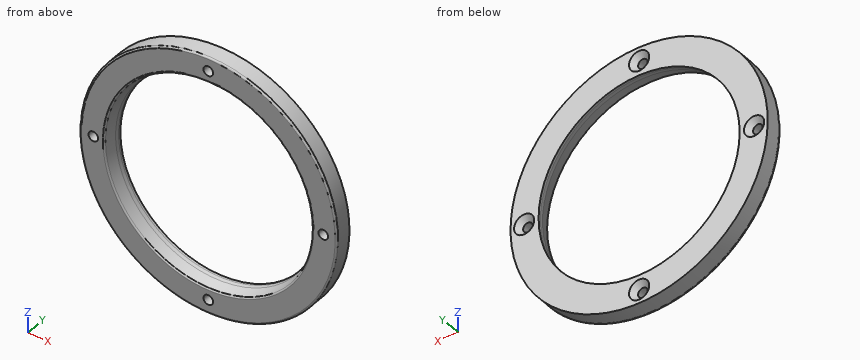
```python
from build123d import *

# Parameters (mm, degrees)
SKETCH1_R                                       = 59.944
SKETCH1_R_2                                     = 47.244
BOSS_EXTRUDE1_DEPTH                             = 8.128
CSK_FOR_M4_FLAT_HEAD_MACHINE_SCREW1_D           = 4.5
CSK_FOR_M4_FLAT_HEAD_MACHINE_SCREW1_CSINK_D     = 9.4
CSK_FOR_M4_FLAT_HEAD_MACHINE_SCREW1_CSINK_ANGLE = 90
CIRPATTERN1_COUNT                               = 4
DRAFT2_ANGLE                                    = 15
SKETCH5_R                                       = 46.865275631
CUT_EXTRUDE1_DEPTH                              = 86.162378173
FILLET1_R                                       = 6.35
FILLET2_R                                       = 0.79375


with BuildPart() as part:
    # Sketch1 → Boss-Extrude1 (new body)
    with BuildSketch(Plane(origin=(0, 0, 0), x_dir=(1, 0, 0), z_dir=(0, 1, 0))):
        with Locations(Location((0, 0, 0), (0, 0, 270))):
            Circle(SKETCH1_R)
        with Locations(Location((0, 0, 0), (0, 0, 270))):
            Circle(SKETCH1_R_2, mode=Mode.SUBTRACT)
    extrude(amount=BOSS_EXTRUDE1_DEPTH)

    # CSK for M4 Flat Head Machine Screw1 (through all)
    with Locations(Plane(origin=(0, 8.128, -53.594), x_dir=(0, 0, 1), z_dir=(0, 1, 0))):
        with Locations((0, 0)):
            csk_for_m4_flat_head_machine_screw1 = CounterSinkHole(CSK_FOR_M4_FLAT_HEAD_MACHINE_SCREW1_D / 2, CSK_FOR_M4_FLAT_HEAD_MACHINE_SCREW1_CSINK_D / 2, counter_sink_angle=CSK_FOR_M4_FLAT_HEAD_MACHINE_SCREW1_CSINK_ANGLE)

    # CirPattern1: CSK for M4 Flat Head Machine Screw1 ×4 about axis
    cirpattern1_axis = Axis((0, 0, 0), (0, 1, 0))
    for i in range(1, CIRPATTERN1_COUNT):
        add(csk_for_m4_flat_head_machine_screw1.rotate(cirpattern1_axis, i * 360 / CIRPATTERN1_COUNT), mode=Mode.SUBTRACT)

    # Draft2
    draft2_faces = [part.faces().sort_by_distance(p)[0] for p in [
        (0, 4.064, -47.244),
    ]]
    draft(draft2_faces, Plane(origin=(0, 0, 0), x_dir=(0, 0, -1), z_dir=(0, -1, 0)), DRAFT2_ANGLE)

    # Sketch4 → Cut-Revolve1 (revolve, cut)
    with BuildSketch(Plane(origin=(0, 0, 0), x_dir=(0, 0, -1), z_dir=(1, 0, 0)), mode=Mode.PRIVATE) as cut_revolve1_sk:
        Polygon((47.244, 0), (45.066108964, 8.128), (46.336108964, 8.128), (48.514, 0), align=None)
    revolve(cut_revolve1_sk.sketch.rotate(Axis((0, 8.128, 0), (0, -1, 0)), 180), axis=Axis((0, 8.128, 0), (0, -1, 0)), mode=Mode.SUBTRACT)

    # Sketch5 → Cut-Extrude1 (cut, through all)
    with BuildSketch(Plane(origin=(0, 8.128, 0), x_dir=(1, 0, 0), z_dir=(0, 1, 0))):
        with Locations(Location((0, 0, 0), (0, 0, 270))):
            Circle(SKETCH5_R)
    extrude(amount=-CUT_EXTRUDE1_DEPTH, mode=Mode.SUBTRACT)

    # Fillet1
    fillet1_edges = [part.edges().sort_by_distance(p)[0] for p in [
        (0, 6.153123114, -46.865275631),
    ]]
    fillet(fillet1_edges, radius=FILLET1_R)

    # Fillet2
    fillet2_edges = [part.edges().sort_by_distance(p)[0] for p in [
        (0, 0, -59.944),
        (0, 0, -48.514),
    ]]
    fillet(fillet2_edges, radius=FILLET2_R)


solid = part.part
```
Can you work these out from the model? Positions are in its coordinate system, mm. Coordinates: 2 decimals unless noted, no trailing zeros.
1) For pin 1 (5 mm diameter, centred on x = -23.5, z = 37.5, fed in from -Y); pin 2 (3 mm diameter, centred on x = 19.5, y = 1, fed in from -Z); pin 3 (4 mm diameter, centred on y = 7, z = 40, fed in from +X); pin 4 (2 mm diameter, centred on x = 26, y = 2.5, fed in from +Z), each with a flat end and sliding along its axis, tell me the tip position at first contact or that it passes through.
2) I need wall thicknesses on probe 1 along X at (y, z) = (1.75, -55); probe 2 along X at (y, z) = (2.75, 53); probe 3 along Z at (x, y) = (7.5, 7). Which ranges of each line are inside material? Lowest first, please.
3) Imagine slicing it at A-A on z = 0. State how many separate pieces and enclosed holes the cut face has, plus the area to 3 significant figures.
Completed:
1. pin 1: passes through
1. pin 2: stops at z = -57.18
1. pin 3: stops at x = 46.36
1. pin 4: stops at z = 54.48
2. probe 1: x = -23.84 to -1.76, 1.76 to 23.84
2. probe 2: x = -28.01 to -2.17, 2.17 to 28.01
2. probe 3: z = -59.47 to -46.26, 46.26 to 59.47
3. separate pieces: 4
3. enclosed holes: 0
3. area: 117 mm2
